Geometry: see drawing. Coordinates: mm, zero at the bounding-box minimum. Coordinates: 2 decimals unless noted, no trailing zeros. Order: outer loops, then holes, each group sorted by start corner. A loop starts at its lowest first (then second) coordinate and runs counter-clockwise, first axis right, second up.
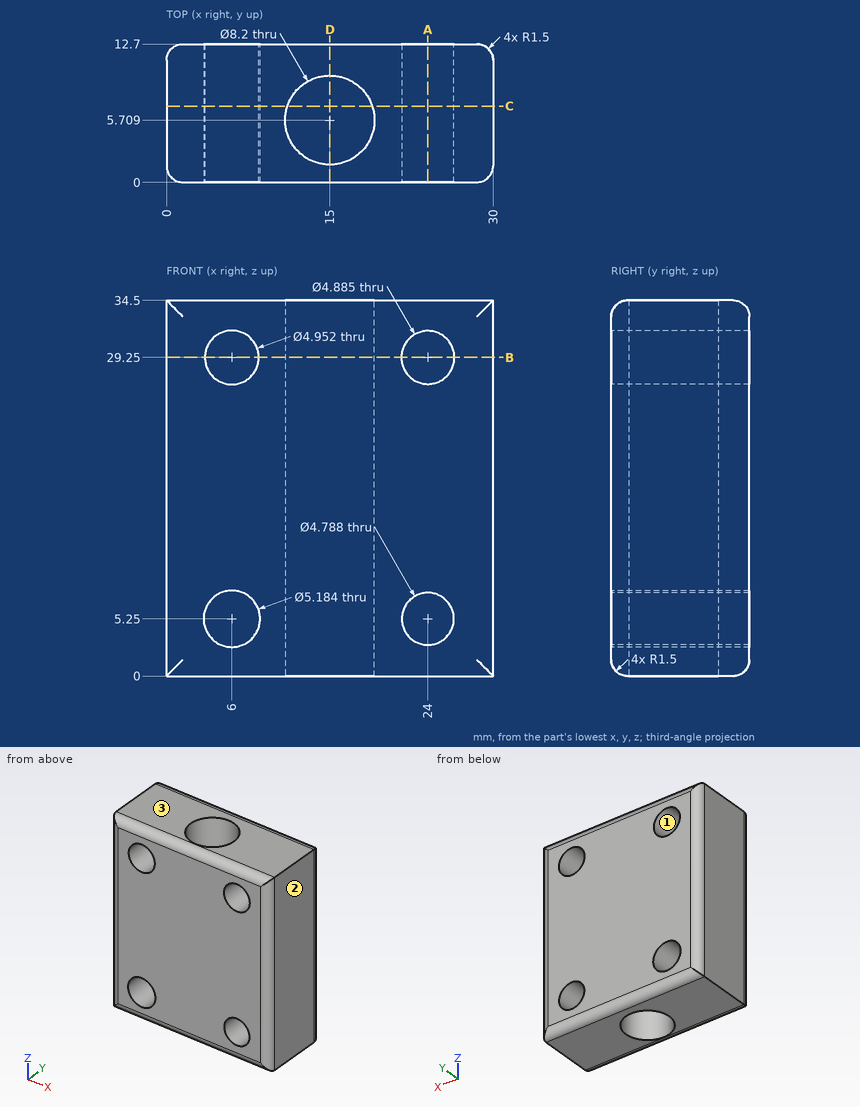
Item 1: Draft query along X for the marked faces 1, 2 and 3. Return one class per face: pulls with the +X half, pulls with the -X half, needs draft (parallel to the pull), parting line crosses it, or undercut.
Response values:
face 1: undercut
face 2: pulls with the +X half
face 3: needs draft
Item 2: Cut plane D-D on x = 15. Return loops of the section in (y, z).
Response values:
outline: (0, 1.5) arc R1.5 ccw to (1.5, 0) - (1.61, 0) - (1.61, 34.5) - (1.5, 34.5) arc R1.5 ccw to (0, 33) - close; (9.81, 0) - (11.2, 0) arc R1.5 ccw to (12.7, 1.5) - (12.7, 33) arc R1.5 ccw to (11.2, 34.5) - (9.81, 34.5) - close
Item 3: Ray query, probe 1 along Z at (x, y) = (6, 6.25) (1 decimal); probe 2 along Z at (x, y) = (24, 6) (1 decimal); probe 3 along Y at (x, z) = (15, 11.5). Return the intervals inside material, ascending.
Response values:
probe 1: z = 0 to 2.7, 7.8 to 26.8, 31.7 to 34.5
probe 2: z = 0 to 2.9, 7.6 to 26.8, 31.7 to 34.5
probe 3: y = 0 to 1.61, 9.81 to 12.7
Item 4: Cut plane B-B on z = 29.25. Return loops of the section in (x, y) (1 decimal).
Response values:
outline: (0, 1.5) arc R1.5 ccw to (1.5, 0) - (3.5, 0) - (3.5, 12.7) - (1.5, 12.7) arc R1.5 ccw to (0, 11.2) - close; (8.5, 0) - (21.6, 0) - (21.6, 12.7) - (8.5, 12.7) - close; (26.4, 0) - (28.5, 0) arc R1.5 ccw to (30, 1.5) - (30, 11.2) arc R1.5 ccw to (28.5, 12.7) - (26.4, 12.7) - close; hole circle Ø8.2 at (15, 5.7)
Item 5: Cut plane A-A on x = 24. Return loops of the section in (y, z) (1 decimal).
Response values:
outline: (0, 1.5) arc R1.5 ccw to (1.5, 0) - (11.2, 0) arc R1.5 ccw to (12.7, 1.5) - (12.7, 2.9) - (0, 2.9) - close; (0, 7.6) - (12.7, 7.6) - (12.7, 26.8) - (0, 26.8) - close; (0, 31.7) - (12.7, 31.7) - (12.7, 33) arc R1.5 ccw to (11.2, 34.5) - (1.5, 34.5) arc R1.5 ccw to (0, 33) - close
Item 6: Cut plane C-C on y = 7. Count the separate pieces of the cut face and the enclosed holes in it.
Response values:
separate pieces: 2
enclosed holes: 4
